from build123d import *

# Parameters (mm, degrees)
SKETCH_1_W          = 30
SKETCH_1_H          = 30
SKETCH_1_W_2        = 26
SKETCH_1_H_2        = 26
EXTRUDE_1_DEPTH     = 100
SKETCH_3_R          = 1.6
CUT_EXTRUDE_1_DEPTH = 106.475115549
SKETCH_5_R          = 1.6
CUT_EXTRUDE_3_DEPTH = 106.475115549
SKETCH_6_R          = 2
CUT_EXTRUDE_4_DEPTH = 106.475115549
SKETCH_7_W          = 17.574392575
SKETCH_7_H          = 17.83033033
SKETCH_7_W_2        = 16.806579307
SKETCH_7_H_2        = 18.854081354
EXTRUDE_2_DEPTH     = 1
CUT_EXTRUDE_5_REACH = 107.475


with BuildPart() as part:
    # 草图1 → 凸台-拉伸1 (new body)
    with BuildSketch(Plane.XY):
        Rectangle(SKETCH_1_W, SKETCH_1_H)
        Rectangle(SKETCH_1_W_2, SKETCH_1_H_2, mode=Mode.SUBTRACT)
    extrude(amount=EXTRUDE_1_DEPTH)

    # 草图3 → 切除-拉伸1 (cut, through all)
    with BuildSketch(Plane(origin=(0, 15, 0), x_dir=(1, 0, 0), z_dir=(0, 1, 0))):
        with Locations(Location((0.5, -94.5, 0), (0, 0, 270))):
            Circle(SKETCH_3_R)
        with Locations(Location((9.5, -94.5, 0), (0, 0, 270))):
            Circle(SKETCH_3_R)
        with Locations(Location((9.5, -85.5, 0), (0, 0, 270))):
            Circle(SKETCH_3_R)
        with Locations(Location((0.5, -85.5, 0), (0, 0, 270))):
            Circle(SKETCH_3_R)
        with Locations(Location((9.5, -14.5, 0), (0, 0, 270))):
            Circle(SKETCH_3_R)
        with Locations(Location((9.5, -5.5, 0), (0, 0, 270))):
            Circle(SKETCH_3_R)
        with Locations(Location((0.5, -5.5, 0), (0, 0, 270))):
            Circle(SKETCH_3_R)
        with Locations(Location((0.5, -14.5, 0), (0, 0, 270))):
            Circle(SKETCH_3_R)
        with Locations(Location((9.5, -70.5, 0), (0, 0, 270))):
            Circle(SKETCH_3_R)
        with Locations(Location((9.5, -61.5, 0), (0, 0, 270))):
            Circle(SKETCH_3_R)
        with Locations(Location((9.5, -38.5, 0), (0, 0, 270))):
            Circle(SKETCH_3_R)
        with Locations(Location((9.5, -29.5, 0), (0, 0, 270))):
            Circle(SKETCH_3_R)
    extrude(amount=-CUT_EXTRUDE_1_DEPTH, mode=Mode.SUBTRACT)

    # 草图5 → 切除-拉伸3 (cut, through all)
    with BuildSketch(Plane(origin=(15, 0, 0), x_dir=(0, 0, -1), z_dir=(1, 0, 0))):
        with Locations(Location((-92.5, -7.5, 0), (0, 0, 90))):
            Circle(SKETCH_5_R)
        with Locations(Location((-7.5, -7.5, 0), (0, 0, 90))):
            Circle(SKETCH_5_R)
    extrude(amount=-CUT_EXTRUDE_3_DEPTH, mode=Mode.SUBTRACT)

    # 草图6 → 切除-拉伸4 (cut, through all)
    with BuildSketch(Plane(origin=(15, 0, 0), x_dir=(0, 0, -1), z_dir=(1, 0, 0))):
        with Locations(Location((-62.5, 5, 0), (0, 0, 90))):
            Circle(SKETCH_6_R)
        with Locations(Location((-37.5, 5, 0), (0, 0, 90))):
            Circle(SKETCH_6_R)
    extrude(amount=-CUT_EXTRUDE_4_DEPTH, mode=Mode.SUBTRACT)

    # 草图7 → 凸台-拉伸2 (add)
    with BuildSketch(Plane.XZ.offset(15)):
        with Locations((4.265629266, 89.627695878)):
            Rectangle(SKETCH_7_W, SKETCH_7_H)
        with Locations((4.6495359, 10.628241878)):
            Rectangle(SKETCH_7_W_2, SKETCH_7_H_2)
    extrude(amount=-EXTRUDE_2_DEPTH)

    # 草图8 → 切除-拉伸5 (cut, up to next)
    with BuildSketch(Plane.XZ.offset(15), mode=Mode.PRIVATE) as cut_extrude_5_sk1:
        with BuildLine():
            Line((14, 70.5), (14, 61.5))
            ThreePointArc((14, 61.5), (9.5, 57), (5, 61.5))
            Line((5, 61.5), (5, 70.5))
            ThreePointArc((5, 70.5), (9.5, 75), (14, 70.5))
        make_face()
    cut_extrude_5_tool1 = extrude(cut_extrude_5_sk1.sketch, amount=-CUT_EXTRUDE_5_REACH, mode=Mode.PRIVATE) & part.part
    # 草图8 → 切除-拉伸5 (cut, up to next)
    with BuildSketch(Plane.XZ.offset(15), mode=Mode.PRIVATE) as cut_extrude_5_sk2:
        with BuildLine():
            Line((14, 29.5), (14, 38.5))
            ThreePointArc((14, 38.5), (9.5, 43), (5, 38.5))
            Line((5, 38.5), (5, 29.5))
            ThreePointArc((5, 29.5), (9.5, 25), (14, 29.5))
        make_face()
    cut_extrude_5_tool2 = extrude(cut_extrude_5_sk2.sketch, amount=-CUT_EXTRUDE_5_REACH, mode=Mode.PRIVATE) & part.part
    add(cut_extrude_5_tool1.solids().sort_by_distance((9.5, -15, 66))[0], mode=Mode.SUBTRACT)
    add(cut_extrude_5_tool2.solids().sort_by_distance((9.5, -15, 34))[0], mode=Mode.SUBTRACT)


solid = part.part
CAD build for the part. Positions are in the model's coordinates, mm. A direction names the side the tool comes from. Round coordinates to 2 decimals unless told otherwise and drop trailing zeros. Write each loop counter-clockwise with the first axis right and the second up, starting at its lowest first coordinate (ties: lowest second). Pieces come first, ordered by that corner, then holes. Notation, with made-up numbers: M 75,-20.75 L 132,-20.75 A18 ccw 132,-1.75 Z; hole C -18.75,58 d2. An arc over 180 degrees is marked long. Put each result on its own line as item: value. Start each with the question number.
1) 3-axis set-ups, long thin cutter, end or side, ignore diameter. For faces 1 (the flat face through (-3, 13, 49)), 2 (the cylindrical face through (8.53, -13.49, 13.23)), 3 (the flat face through (5, 14, 66)), 4 (the cylindrical face through (14.451, 6.075, 39.186)): which of +Z, -Z, +X, -X, +Y, -Y reach the whole face in a straight line?
2) Drill centre lines: probe 1 along Z at (x, y) = (-13.85, -7.5); probe 2 along X at (y, z) = (11, 53.5); probe 3 along Y at (x, z) = (-13.6, 92.5). Where is each one in solid material? Low to high. Write a range as [from, to].
3) Pin check, flat tip, straight feed: pin 1 Ø1.9 at (x, z) = (0.5, 5.5) entering from +Y. Stop position of the tip, or through.
4) Pull direction X, two halves, no side cores. Call faces 5 (the cylindrical face through (14.014, -7.708, 94.086)), 6 (the cylindrical face through (8.53, 14.01, 84.23)): pulls with the +X half, pulls with the -X half, needs draft (parallel to the pull), parting line crosses it, or undercut.
5) Saw through at D-D, the plane z = 52.5. Write the cut outline in (x, y), and give its area (3 significant figures).
6) Saw through at A-A, the plane x = -10.5. Write the cut outline in (y, z), and give its area (3 significant figures).
7) Saw through at C-C, the plane z = 62.5. Write the cut outline in (x, y).
8) Saw through at B-B, the plane y = 5. Count the separate pieces of the cut face and the enclosed holes in it, and give its area (3 significant figures).
Resolved:
1. face 1: +Z, -Z
1. face 2: +Y
1. face 3: +Y, -Y
1. face 4: +X, -X
2. probe 1: [0, 5.9], [9.1, 90.9], [94.1, 100]
2. probe 2: [-15, -13], [13, 15]
2. probe 3: [-15, -9.1], [-5.9, 15]
3. pin 1: y = -14
4. face 5: needs draft
4. face 6: undercut
5. outline: M -15,-15 L 15,-15 L 15,15 L -15,15 Z; hole M -13,-13 L 13,-13 L 13,13 L -13,13 Z
5. area: 224 mm²
6. outline: M -15,0 L -13,0 L -13,100 L -15,100 Z; M 13,0 L 15,0 L 15,100 L 13,100 Z
6. area: 400 mm²
7. outline: M -15,-15 L 5,-15 L 5,-13 L -13,-13 L -13,3 L -15,3 Z; M -15,7 L -13,7 L -13,13 L 5,13 L 5,15 L -15,15 Z; M 14,-15 L 15,-15 L 15,3 L 14,3 Z; M 14,7 L 15,7 L 15,15 L 14,15 Z
8. separate pieces: 6
8. enclosed holes: 0
8. area: 350 mm²
